CAD build for the part. Positions are in the model's coordinates, mm. A direction names the side the tool comes from. Coordinates: 2 decimals unless noted, no trailing zeros. Loops run counter-clockwise (first coordinate to the right, second up) from the corner with the lowest first, then second, coordinate; pieces in that order, holes last.
1) Pin check, flat tips, straight feed: pin 1 Ø1 at (x, z) = (4, -7) entering from +Y; pin 2 Ø0.6 at (y, z) = (5, -4.5) entering from -X; pin 3 Ø3 at (y, z) = (4, 4) entering from +X. Stop position of each tip, or through.
2) Wall check: line 1 along X through (y, z) = (2.2, 6.44); line 2 along X through (y, z) = (2.75, -6.26); line 3 along Z through (x, y) = (28.5, 1.75). Give the ranges that are in metal, low to high.
3) Two-plate mould, pull along Z, no slides. Class faces 1 (the cylindrical face through (19.043, 2.028, 5.989)), 2 (the cylindrical face through (46.13, 0.47, -9.5)), 3 (the flat face through (21.25, -1, -6)): +Z half, -Z half, draft (parallel to the pull), parting line (faces both ways), or undercut.
4) Which spindle directions (+Z, -Z, +X, -X, +Y, -Y) get a long thin tool onto all of the face, cutting with end or side? Do faces 4 (the flat face through (0, 2, -10.25)), 5 (the flat face through (0, 0, 0)), 6 (the flat face through (0, 4, 0)). Say none if no direction does.
5) Saw through at A-A, the plane z = 6.44. Write the cut outline in (x, y).
6) Saw through at C-C, the plane y = 2. Give the number of separate pieces and of enclosed holes in the cut face, and give its area (3 significant figures).
7) Saw through at B-B, the plane x = 67. Write the cut outline in (y, z).
```python
from build123d import *

# Parameters (mm, degrees)
SKETCH1_W           = 42.5
SKETCH1_H           = 20.5
BOSS_EXTRUDE1_DEPTH = 4
SKETCH2_R           = 4
BOSS_EXTRUDE2_DEPTH = 53
FILLET1_R           = 2.54
SKETCH4_R           = 1.5
CUT_EXTRUDE2_DEPTH  = 7.0000001


with BuildPart() as part:
    # Sketch1 → Boss-Extrude1 (new body)
    with BuildSketch(Plane(origin=(0, 0, 0), x_dir=(1, 0, 0), z_dir=(0, 1, 0))):
        Rectangle(SKETCH1_W, SKETCH1_H)
    extrude(amount=BOSS_EXTRUDE1_DEPTH)

    # Sketch2 → Boss-Extrude2 (add)
    with BuildSketch(Plane(origin=(21.25, 0, 0), x_dir=(0, 0, -1), z_dir=(1, 0, 0))):
        with Locations((5.804410425, 2)):
            Circle(SKETCH2_R)
    extrude(amount=BOSS_EXTRUDE2_DEPTH)

    # Fillet1
    fillet1_edges = [part.edges().sort_by_distance(p)[0] for p in [
        (74.25, 2, -1.804410425),
    ]]
    fillet(fillet1_edges, radius=FILLET1_R)

    # Sketch4 → Cut-Extrude2 (cut, through all)
    with BuildSketch(Plane(origin=(0, 4, 0), x_dir=(1, 0, 0), z_dir=(0, 1, 0))):
        with Locations((17.612, -6.44)):
            Circle(SKETCH4_R)
        with Locations((-7.788, 6.26)):
            Circle(SKETCH4_R)
    extrude(amount=-CUT_EXTRUDE2_DEPTH, mode=Mode.SUBTRACT)


solid = part.part
```
Data:
1. pin 1: stops at y = 4
1. pin 2: stops at x = 21.25
1. pin 3: stops at x = 21.25
2. line 1: x = -21.25 to 16.11, 19.11 to 21.25
2. line 2: x = -21.25 to -9.29, -6.29 to 74.25
2. line 3: z = -9.8 to -1.81
3. face 1: undercut
3. face 2: parting line
3. face 3: draft
4. face 4: -Z, +X, -X, +Y, -Y
4. face 5: +Z, -Z, -X, -Y
4. face 6: +Z, -Z, -X, +Y
5. outline: (-21.25, 0) - (16.11, 0) - (16.11, 4) - (-21.25, 4) - close; (19.11, 0) - (21.25, 0) - (21.25, 4) - (19.11, 4) - close
6. separate pieces: 1
6. enclosed holes: 2
6. area: 1,280 mm2
7. outline: circle Ø8 at (2, -5.8)
